from build123d import *

# Parameters (mm, degrees)
F0_W     = 26.9435550738
F0_H     = 11.2643459439
F0_H_2   = 7.4713081121
F0_W_2   = 6.1128898524
F1_DEPTH = 35
F0_H_3   = 23.3753739297
F0_W_3   = 14.827863574
F2_DEPTH = 5
F3_W     = 44
F3_H     = 23
F4_DEPTH = 30
F6_DEPTH = 25


with BuildPart() as f1:
    # F0 (on Top) → F1 (new body)
    with BuildSketch(Plane.XY):
        with Locations((16.5282224631, 9.367827028)):
            Rectangle(F0_W, F0_H)
        with Locations((16.5282224631, -9.367827028)):
            Rectangle(F0_W, F0_H)
        with Locations((16.5282224631, 0)):
            Rectangle(F0_W, F0_H_2)
        with Locations((-16.5282224631, 9.367827028)):
            Rectangle(F0_W, F0_H)
        with Locations((-16.5282224631, 0)):
            Rectangle(F0_W, F0_H_2)
        with Locations((-16.5282224631, -9.367827028)):
            Rectangle(F0_W, F0_H)
        with Locations((0, -9.367827028)):
            Rectangle(F0_W_2, F0_H)
        Rectangle(F0_W_2, F0_H_2)
        with Locations((0, 9.367827028)):
            Rectangle(F0_W_2, F0_H)
    extrude(amount=F1_DEPTH)

    # F0 (on Top) → F2 (join)
    with BuildSketch(Plane.XY):
        with Locations((0, 26.6876869649)):
            Rectangle(F0_W_2, F0_H_3)
        with Locations((37.413931787, 0)):
            Rectangle(F0_W_3, F0_H_2)
        with Locations((-37.413931787, 0)):
            Rectangle(F0_W_3, F0_H_2)
        with Locations((0, -26.6876869649)):
            Rectangle(F0_W_2, F0_H_3)
    extrude(amount=F2_DEPTH)

    # F3 (on face) → F4 (cut)
    with BuildSketch(Plane.XY.offset(35)):
        Rectangle(F3_W, F3_H)
    extrude(amount=-F4_DEPTH, mode=Mode.SUBTRACT)

    # F5 (on face) → F6 (cut)
    with BuildSketch(Plane.YZ.offset(-22)):
        Polygon((-4.0054083802, 5), (0, 5), (0, 7.6920529827), (0, 10.3841059655), (-4.0054083802, 10.3841059655), align=None)
        Polygon((0, 7.6920529827), (0, 5), (4.0054083802, 5), (4.0054083802, 10.3841059655), (0, 10.3841059655), align=None)
    extrude(amount=-F6_DEPTH, mode=Mode.SUBTRACT)


solid = f1.part
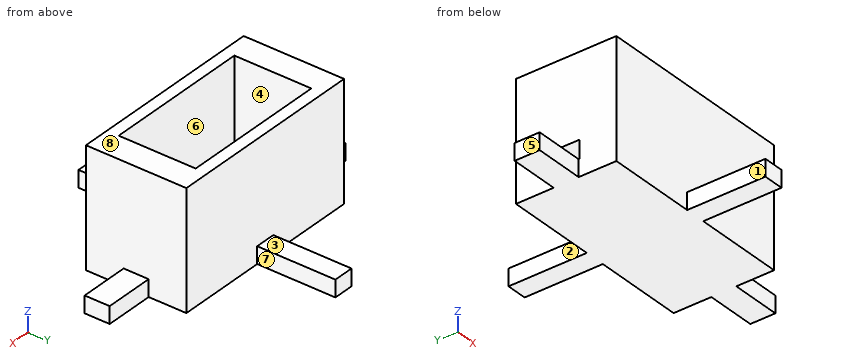
Work out the finished part from the listing and answer in its coordinate system (mm). Face numbers are marked on the shaded views. A direction names the side the tool comes from. Round coordinates to 2 decimals unless told otherwise and drop trailing zeros. Loops run counter-clockwise (first coordinate to the right, second up) from the corner with the lowest first, then second, coordinate; pieces in that order, holes last. Notation, with made-up numbers: M 78.5,27.5 L 95.5,27.5 A20 cw 95.5,48.5 Z; hole C 75.5,-16.5 d2. An arc over 180 degrees is marked long. One line per question, with ' | ' between items. Start each with the question number.
(1) A cutting plane is placed at B-B on y = 2.5. Write down the section's boundary in (x, z).
(2) For a pull along X with two mould halves and no side action, classify the marked faces 5, 6, 7 and 8 as released by +X, released by -X, zero draft, split by the parting line, or undercut.
(3) A cutting plane is placed at C-C on x = -27.5. Write down the section's boundary in (y, z).
(4) Flat-ended cylindrical pins translate along their axes: pin 1 Ø5.5 at (x, z) = (-39, 3) entering from -Y; pin 2 Ø3 at (y, z) = (11.5, 24.5) entering from +X; pin 3 Ø3 at (x, z) = (-23.5, 11) entering from +Y; pin 4 Ø4 at (x, y) = (-27.5, -1) entering from -Z. Find the tip coordinate at first contact, or state that the pin passes through.
(5) Find the intervals of material crossed by line 1 (Y direction, x = -0.5, z = 20.5); line 2 (X direction, y = -1, z = 28); line 3 (X direction, y = 3.5, z = 8), in increasing order.
(6) A tool of negligible diameter and unlimited length cuts with its end or side. For the marked faces 1, 2, 3 and 4, from which of +Z, -Z, +X, -X, +Y, -Y can it reach the whole face along a straight path? Write none if from no direction.
(7) A cutting plane is placed at D-D on x = -2. Write down the section's boundary in (y, z).
(8) A cutting plane is placed at A-A on z = 22.5. Write down the section's boundary in (x, y).
Geometry check:
1) outline: M -44.83,0 L 44.83,0 L 44.83,5 L 30,5 L 30,35 L 22,35 L 22,5 L -44.83,5 Z; M -30,10.38 L -22,10.38 L -22,35 L -30,35 Z
2) face 5: released by -X | face 6: undercut | face 7: released by +X | face 8: zero draft
3) outline: M -15,0 L 15,0 L 15,35 L -15,35 Z; hole M -4.01,5 L 4.01,5 L 4.01,10.38 L -4.01,10.38 Z
4) pin 1: stops at y = -3.74 | pin 2: stops at x = 30 | pin 3: stops at y = 15 | pin 4: stops at z = 0
5) line 1: y = -15 to -11.5, 11.5 to 15 | line 2: x = -30 to -22, 22 to 30 | line 3: x = 22 to 30
6) face 1: +Z, -Z, -X, -Y | face 2: +Z, -Z, -X, +Y | face 3: +Z, +X, -X, +Y | face 4: +Z
7) outline: M -38.38,0 L 38.38,0 L 38.38,5 L 15,5 L 15,35 L 11.5,35 L 11.5,5 L -11.5,5 L -11.5,35 L -15,35 L -15,5 L -38.38,5 Z
8) outline: M -30,-15 L 30,-15 L 30,15 L -30,15 Z; hole M -22,-11.5 L 22,-11.5 L 22,11.5 L -22,11.5 Z
